Input: part model. Units: mm. Frame: model coordinates. Face numbers are marked on the shaded views. A direction names the side the tool comes from. Round coordinates to 2 decimals unless told otherwise and drop trailing zeros. Loops run counter-clockwise (first coordinate to the right, second up) from the corner with the lowest first, then second, coordinate; pieces in that order, holes last. Notation, with made-up numbers: (60.25, 21) -> (77.25, 21) arc R29 cw to (77.25, 60) -> close; hole circle Ø10 at (72, 67). An arc over 180 degrees is marked (long way). Answer as a JSON object with one key per item and string values. Group by question number.
Item 1: Section query C-C on x = 55. Return loops of the section in (y, z), and give its area (3 significant figures).
Item 2: Section query A-A on z = -17.5. Return loops of the section in (x, y).
Item 3: Section query D-D on y = 11. Count the separate pieces of the cut face and the enclosed holes in it, and give its area (3 significant figures).
Item 4: Pin query (flat end, axial travel): pin 1 (6 mm diameter, centred on x = -29.5, z = 29, fed in from -Y); pin 2 (12 mm diameter, centred on x = 3, z = -24.5, fed in from +Y); pin 3 (22 mm diameter, centred on x = -72, y = 49, fed in from +Z). Return the tip coordinate at first contact, or that it passes through.
Item 5: Draft query along X for the marked faces 5, 6, 7 and 8. Return one class per face: released by +X, released by -X, zero draft, split by the parting line, or undercut.
Item 6: Material intervals for line 1 (X direction, y = 6.25, z = -25); line 2 (Z direction, x = 44, y = 12.5); line 3 (Z direction, x = 46, y = 13), sorted ascending. Write a range as [from, to].
Item 7: Set-up query: the marked faces 1, 2, 3 and 4. Return all of +Z, -Z, +X, -X, +Y, -Y with unobstructed straight access to the full face (end or side cutting, diameter ignored); none if empty.
Item 8: Section query B-B on x = -86.5. Return loops of the section in (y, z).
from build123d import *

# Parameters (mm, degrees)
SKETCH1_W           = 150
SKETCH1_H           = 100
BOSS_EXTRUDE1_DEPTH = 25
SKETCH2_W           = 100
SKETCH2_H           = 90
BOSS_EXTRUDE2_DEPTH = 25
FILLET1_R           = 25
BOSS_EXTRUDE3_REACH = 196.068
SKETCH5_W           = 80
SKETCH5_H           = 102.358362639
SKETCH6_W           = 80
SKETCH6_H           = 15
CUT_EXTRUDE1_DEPTH  = 15
SKETCH7_R           = 15
CUT_EXTRUDE2_DEPTH  = 195.068286951
SKETCH8_R           = 10
CUT_EXTRUDE3_DEPTH  = 144.527000944
SKETCH9_R           = 10
CUT_EXTRUDE4_DEPTH  = 207.415919487
FILLET4_R           = 40


with BuildPart() as part:
    # Sketch1 → Boss-Extrude1 (new body)
    with BuildSketch(Plane(origin=(0, 0, 0), x_dir=(1, 0, 0), z_dir=(0, 1, 0))):
        Rectangle(SKETCH1_W, SKETCH1_H)
    extrude(amount=BOSS_EXTRUDE1_DEPTH)

    # Sketch2 → Boss-Extrude2 (add)
    with BuildSketch(Plane.ZY.offset(75)):
        with Locations((0, -20)):
            Rectangle(SKETCH2_W, SKETCH2_H)
    extrude(amount=BOSS_EXTRUDE2_DEPTH)

    # Fillet1
    fillet1_edges = [part.edges().sort_by_distance(p)[0] for p in [
        (-87.5, -65, -50),
        (-87.5, -65, 50),
        (75, 12.5, 50),
        (75, 12.5, -50),
    ]]
    fillet(fillet1_edges, radius=FILLET1_R)

    # Sketch5 → Boss-Extrude3 (add, up to next)
    with BuildSketch(Plane(origin=(-62.5, 62.5, 0), x_dir=(0, 0, -1), z_dir=(0.7071067811865438, -0.7071067811865512, 0)), mode=Mode.PRIVATE) as boss_extrude3_sk1:
        with Locations((0, -1.85382727)):
            Rectangle(SKETCH5_W, SKETCH5_H)
    boss_extrude3_tool1 = extrude(boss_extrude3_sk1.sketch, amount=BOSS_EXTRUDE3_REACH, mode=Mode.PRIVATE) - part.part
    add(boss_extrude3_tool1.solids().sort_by_distance((-63.810854, 61.189146, 0))[0])

    # Sketch6 → Cut-Extrude1 (cut)
    with BuildSketch(Plane(origin=(-62.5, 62.5, 0), x_dir=(0, 0, 1), z_dir=(-0.7071067811865438, 0.7071067811865513, 0))):
        with Locations((0, -20.533008589)):
            Rectangle(SKETCH6_W, SKETCH6_H)
    extrude(amount=-CUT_EXTRUDE1_DEPTH, mode=Mode.SUBTRACT)

    # Sketch7 → Cut-Extrude2 (cut, through all)
    with BuildSketch(Plane(origin=(-62.5, 62.5, 0), x_dir=(0.7071067811865513, 0.7071067811865438, 0), z_dir=(-0.7071067811865438, 0.7071067811865513, 0))):
        with Locations(Location((21.966991411, 0, 0), (0, 0, 180))):
            Circle(SKETCH7_R)
    extrude(amount=-CUT_EXTRUDE2_DEPTH, mode=Mode.SUBTRACT)

    # Sketch8 → Cut-Extrude3 (cut, through all)
    with BuildSketch(Plane(origin=(0, 25, 0), x_dir=(1, 0, 0), z_dir=(0, 1, 0))):
        with Locations(Location((50, 25, 0), (0, 0, 270))):
            Circle(SKETCH8_R)
        with Locations(Location((50, -25, 0), (0, 0, 270))):
            Circle(SKETCH8_R)
    extrude(amount=-CUT_EXTRUDE3_DEPTH, mode=Mode.SUBTRACT)

    # Sketch9 → Cut-Extrude4 (cut, through all)
    with BuildSketch(Plane.ZY.offset(100)):
        with Locations((-25, -40)):
            Circle(SKETCH9_R)
        with Locations((25, -40)):
            Circle(SKETCH9_R)
    extrude(amount=-CUT_EXTRUDE4_DEPTH, mode=Mode.SUBTRACT)

    # Fillet4
    # the kernel refuses this fillet: 40 mm, written as the material it takes off along each edge
    with BuildSketch(Plane(origin=(-98.332385785, 168.088970452, -40), x_dir=(-0.7071067811865511, -0.7071067811865437, 0), z_dir=(0.7071067811865438, -0.7071067811865512, 0))) as fillet4_piece_1_section:
        with BuildLine():
            CenterArc((FILLET4_R, -FILLET4_R), FILLET4_R, 90, 90)
            Line((0, -FILLET4_R), (0, 0))
            Line((0, 0), (FILLET4_R, 0))
        make_face()
    fillet4_piece_1 = extrude(amount=302.358362639, mode=Mode.PRIVATE)
    fillet4_piece_1 = split(fillet4_piece_1, bisect_by=Plane(origin=(-0.418025546, 25, -30.730970788), z_dir=(0, 1, 0)), keep=Keep.TOP, mode=Mode.PRIVATE)
    add(fillet4_piece_1, mode=Mode.SUBTRACT)
    with BuildSketch(Plane(origin=(-98.332385785, 168.088970452, 40), x_dir=(0, 0, -1), z_dir=(0.7071067811865438, -0.7071067811865512, 0))) as fillet4_piece_2_section:
        with BuildLine():
            CenterArc((FILLET4_R, -FILLET4_R), FILLET4_R, 90, 90)
            Line((0, -FILLET4_R), (0, 0))
            Line((0, 0), (FILLET4_R, 0))
        make_face()
    fillet4_piece_2 = extrude(amount=302.358362639, mode=Mode.PRIVATE)
    fillet4_piece_2 = split(fillet4_piece_2, bisect_by=Plane(origin=(-0.418025546, 25, 30.730970789), z_dir=(0, 1, 0)), keep=Keep.TOP, mode=Mode.PRIVATE)
    add(fillet4_piece_2, mode=Mode.SUBTRACT)


solid = part.part
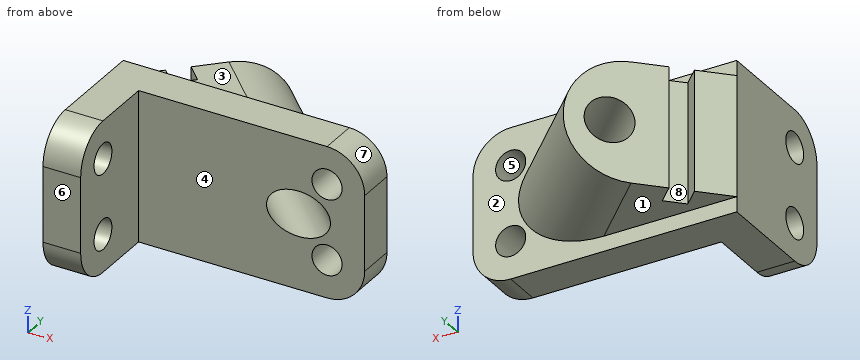
Solved:
{
 "1": {"outline": "(0, -49.49) -> (25, -49.49) -> (25, -33.66) -> (0, -33.66) -> close; (0, -16.34) -> (25, -16.34) -> (25, 16.34) -> (0, 16.34) -> close; (0, 33.66) -> (25, 33.66) -> (25, 49.49) -> (0, 49.49) -> close", "area": "1,610 mm²"},
 "2": {"outline": "(-100, -65) -> (-75, -65) -> (-75, -46.61) -> (-100, -46.61) -> close; (-100, -33.39) -> (-75, -33.39) -> (-75, 0) -> (43.39, 0) -> (43.39, 25) -> (39.06, 25) -> (-30.47, 94.53) -> (-71.72, 53.28) -> (-61.11, 42.68) -> (-71.72, 32.07) -> (-82.32, 42.68) -> (-100, 25) -> close; (56.61, 0) -> (75, 0) -> (75, 25) -> (56.61, 25) -> close"},
 "3": {"separate pieces": "1", "enclosed holes": "3", "area": "15,600 mm²"},
 "4": {"pin 1": "y = 0", "pin 2": "y = 63.24", "pin 3": "z = 40"},
 "5": {"face 5": "undercut", "face 6": "zero draft", "face 7": "released by +X", "face 8": "undercut"},
 "6": {"line 1": "[-100, 40], [60, 75]", "line 2": "[-50, -33], [-17, 17], [33, 50]", "line 3": "[-50, -34.17], [-15.83, 15.83], [34.17, 50]"},
 "7": {"face 1": "-Z, +X, -X, +Y", "face 2": "+X, +Y", "face 3": "+Z, +X, -X, +Y", "face 4": "+Z, -Z, +X, -Y"},
 "8": {"outline": "(-65, -25) arc R25 ccw to (-40, -50) -> (25, -50) -> (25, -40) -> (38.5, -40) -> (38.5, 40) -> (25, 40) -> (25, 50) -> (-40, 50) arc R25 ccw to (-65, 25) -> close; hole circle Ø20 at (-40, -25); hole circle Ø20 at (-40, 25)"}
}
